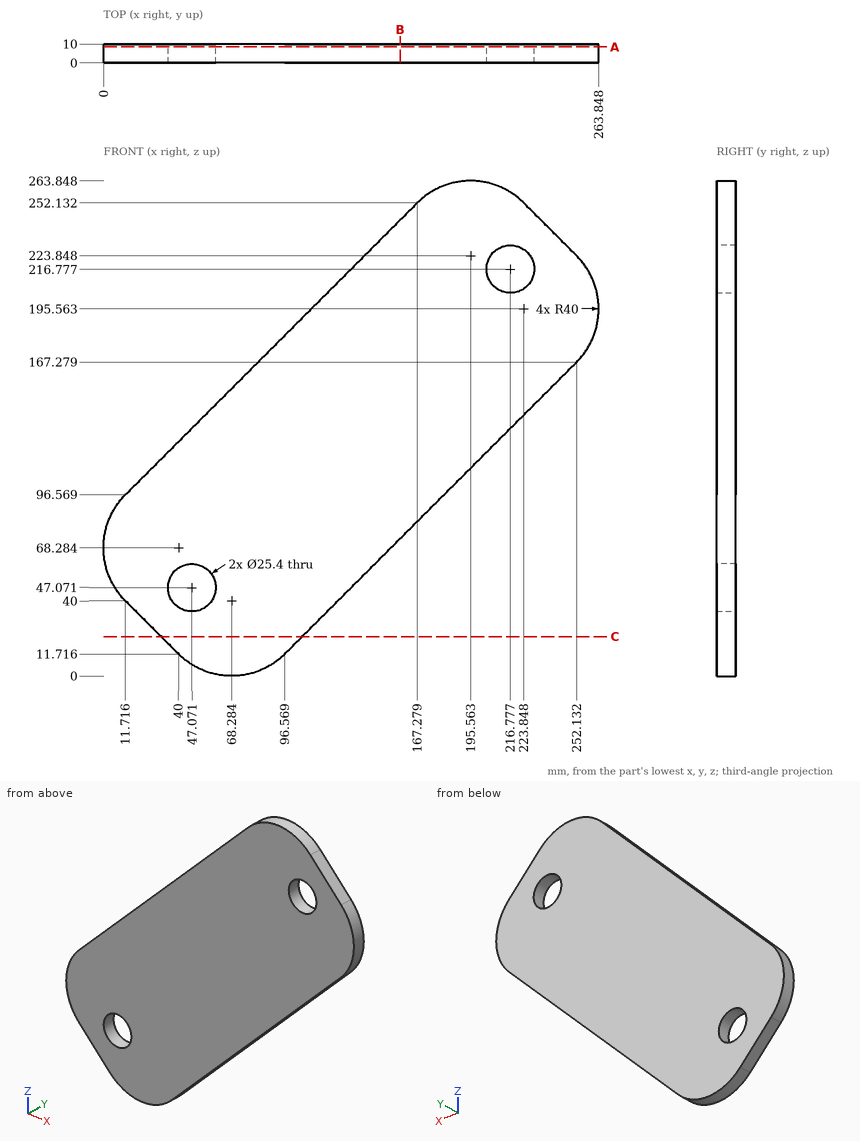
The drawing under review shows one solid part. Ordinate dimensions are in mm from its lowest x, y, z. Round coordinates to 2 decimals unless told otherwise and drop trailing zeros. Order: outer loops, then holes, each group sorted by start corner. A loop starts at its lowest first (then second) coordinate and runs counter-clockwise, first axis right, second up. Notation, with made-up numbers: M 25.25,15.5 L 31.25,15.5 A28 ccw 31.25,43.5 Z; hole C 11.5,-29.5 d11. An arc over 180 degrees is marked long. Answer as CSV lines item,"result". Start each with the question number.
1) Add section B-B (x = 158). Give the boundary of the cut face in (y, z).
2) Add section A-A (y = 8.5). Give the boundary of the cut face in (x, z) (1 decimal), then the cut area to 3 significant figures.
3) Add section C-C (z = 21). Give the boundary of the cut face in (x, y) (1 decimal).
4) For pin 1 Ø5 at (x, y) = (230, 3.5) entering from +Z; pin 2 Ø6 at (x, y) = (193, 1) entering from +Z; pin 3 Ø3 at (x, y) = (111.5, 2.5) entering from -Z, all flat-tipped, find the tip position at first contact; note any pin that passes through.
Resolved:
1,outline,"M 0,73.15 L 10,73.15 L 10,242.85 L 0,242.85 Z"
2,outline,"M 11.7,40 L 40,11.7 A40 ccw 96.6,11.7 L 252.1,167.3 A40 ccw 252.1,223.8 L 223.8,252.1 A40 ccw 167.3,252.1 L 11.7,96.6 A40 ccw Z; hole C 47.1,47.1 d25.4; hole C 216.8,216.8 d25.4"
2,area,"33,600 mm^2"
3,outline,"M 30.7,0 L 105.9,0 L 105.9,10 L 30.7,10 Z"
4,pin 1,"z = 248.48"
4,pin 2,"z = 263.85"
4,pin 3,"z = 25.15"
